from build123d import *

# Parameters (mm, degrees)
F0_R      = 3.7
F0_R_2    = 2.7
F1_DEPTH  = 35
F2_W      = 2
F2_H      = 6.1218521535
F3_DEPTH  = 35.001
F6_W      = 26.1
F6_H      = 2
F8_W      = 26.1
F8_H      = 2
F11_DEPTH = 1.7
F13_DEPTH = 1.7
F14_R     = 6.1
F15_DEPTH = 19.2330509442
F14_R_2   = 8.1
F16_DEPTH = 0.5
F17_R     = 0.49999
F19_DEPTH = 26.1
F21_DEPTH = 1.7
F23_DEPTH = 1.7


# Not quite as in the source:
# - a fillet or chamfer is up to 0.001 mm smaller than in the source, because OpenCascade refuses the exact size


with BuildPart() as f1:
    # F0 (on Top) → F1 (new body)
    with BuildSketch(Plane.XY):
        with Locations((-15.75, 0)):
            Circle(F0_R)
        with Locations((-15.75, 0)):
            Circle(F0_R_2, mode=Mode.SUBTRACT)
    extrude(amount=F1_DEPTH)

    # F2 (on Top) → F3 (cut, through all)
    with BuildSketch(Plane.XY):
        with Locations((-15.75, 2.7)):
            Rectangle(F2_W, F2_H)
    extrude(amount=F3_DEPTH, mode=Mode.SUBTRACT)


with BuildPart() as f5_1:
    # F5: instance of F1
    add(f1.part.mirror(Plane.YZ))


with BuildPart() as f1_1:
    add(f1.part)

    add(f5_1.part)  # F9 merges F5_1
    # F6 (on Top) → F9 section 0
    with BuildSketch(Plane.XY):
        with Locations((0, -10)):
            Rectangle(F6_W, F6_H)
    # F8 (on offset) → F9 section 1
    with BuildSketch(Plane.XY.offset(35)):
        with Locations((0, 10.2072594216)):
            Rectangle(F8_W, F8_H)
    loft()

    # F10 (on face) → F11 (join, through all)
    with BuildSketch(Plane.YZ.offset(13.05)):
        Polygon((2.5079872408, 19.9324185939), (2.5298221281, 19.9702377282), (11.2072594216, 35), (2.5079872408, 35), align=None)
    extrude(amount=F11_DEPTH)

    # F12 (on face) → F13 (join, through all)
    with BuildSketch(Plane(origin=(-13.05, 0, 0), x_dir=(0, -1, 0), z_dir=(-1, 0, 0))):
        Polygon((-11.2072594216, 35), (-2.5298221281, 19.9702377282), (-2.5079872408, 19.9324185939), (-2.5079872408, 35), align=None)
    extrude(amount=F13_DEPTH)

    # F14 (on face) → F15 (cut, through all)
    with BuildSketch(Plane(origin=(0, -8.25, 4.7631397208), x_dir=(1, 0, 0), z_dir=(0, -0.8660254038, 0.5))):
        with Locations((0, 16.5)):
            Circle(F14_R)
    extrude(amount=-F15_DEPTH, mode=Mode.SUBTRACT)

    # F14 (on face) → F16 (join)
    with BuildSketch(Plane(origin=(0, -8.25, 4.7631397208), x_dir=(1, 0, 0), z_dir=(0, -0.8660254038, 0.5))):
        with Locations((0, 16.5)):
            Circle(F14_R_2)
        with Locations((0, 16.5)):
            Circle(F14_R, mode=Mode.SUBTRACT)
    extrude(amount=F16_DEPTH)

    # F17 (radius 0.5 in the source; OpenCascade refuses exactly that, so slightly less here)
    f17_edges = [f1_1.edges().sort_by_distance(p)[0] for p in [
        (-8.1, -0.433013, 19.302559),
    ]]
    fillet(f17_edges, radius=F17_R)

    # F18 (on face) → F19 (cut, through all)
    with BuildSketch(Plane.YZ.offset(13.05)):
        Polygon((-5.3, 9.8726896031), (-11, 0), (-9, 0), (-5.3, 6.408587988), align=None)
    extrude(amount=-F19_DEPTH, mode=Mode.SUBTRACT)

    # F20 (on face) → F21 (join, through all)
    with BuildSketch(Plane.YZ.offset(13.05)):
        Polygon((-2.5298221281, 14.6707784232), (-5.3, 9.8726896031), (-5.3, 6.408587988), (-2.5298221281, 6.408587988), align=None)
    extrude(amount=F21_DEPTH)

    # F22 (on face) → F23 (join, through all)
    with BuildSketch(Plane(origin=(-13.05, 0, 0), x_dir=(0, -1, 0), z_dir=(-1, 0, 0))):
        Polygon((5.3, 6.408587988), (5.3, 9.8726896031), (2.5298221281, 14.6707784232), (2.5298221281, 6.408587988), align=None)
    extrude(amount=F23_DEPTH)


solid = f1_1.part
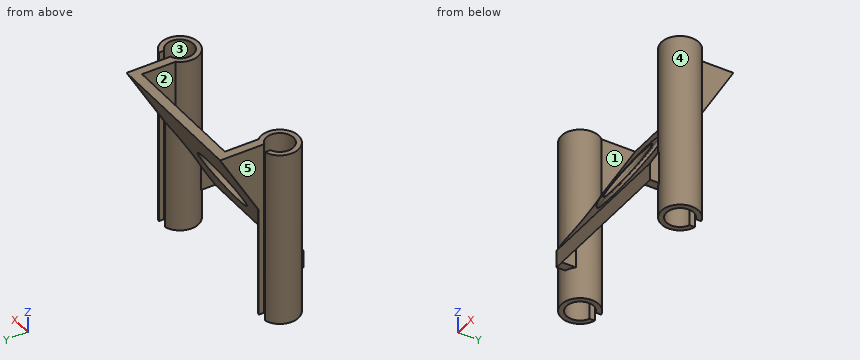
Verification items for the finished model (mm, model axes). Face numbers are marked on the shaded views. A direction names the side the tool comes from. Give positions to 0.01 mm unless a question says otherwise; leave off trailing zeros. Write each loop counter-clockwise with the first axis right and the second up, starting at its lowest first coordinate (ties: lowest second). Pieces come first, ordered by that corner, then holes.
(1) Cross-section at A-A (x = 15.75). Enter the section's corners in (y, z), plus the area to 3 significant figures.
(2) Access from +Z, -Z, +X, -X, +Y, -Y to the whole of each face (thin tool, end or side, straight path). Record for the marked faces 3, 4 and 5.
(3) Cross-section at D-D (x = 10). Enter the section's corners in (y, z), plus the area to 3 significant figures.
(4) Cross-section at B-B (y = 7). Enter the section's corners in (x, z).
(5) Gauge pin test, flat ends, axial feed: pin 1 (5 mm diameter, centred on y = 2, z = 26.5, fed in from -X); pin 2 (0.5 mm diameter, centred on y = -4.5, z = 9.5, fed in from -X); pin 3 (8 mm diameter, centred on x = 1.5, y = 0.5, fed in from -Z); pin 4 (5.5 mm diameter, centred on y = 6, z = 28, fed in from -X). Record the tip position at first contact, or that the pin passes through.
(6) Cross-section at C-C (y = 2). State how many separate pieces and enclosed holes the cut face has, plus the area to 3 significant figures.
(7) Material ranges on line 1 (X direction, y = 0, z = 24); line 2 (X direction, y = 2, z = 24); line 3 (Y direction, x = -14.5, z = 29), recorded low to high.
(8) Mould release check, pull along X, two halves, no side actions. Record for the marked faces 1 and 2: +X half, -X half, draft (parallel to the pull), parting line (faces both ways), or undercut.
Worked out:
1. outline: (-3.7, 0) - (-2.7, 0) - (-2.7, 35) - (-3.7, 35) - close
1. area: 35.0 mm2
2. face 3: +Z, -Z
2. face 4: none
2. face 5: +Z, -Z, +Y
3. outline: (-5.3, 6.41) - (11.21, 35) - (9.21, 35) - (-5.3, 9.87) - close
3. area: 53.7 mm2
4. outline: (-14.75, 27.71) - (14.75, 27.71) - (14.75, 35) - (13.05, 35) - (13.05, 31.18) - (-13.05, 31.18) - (-13.05, 35) - (-14.75, 35) - close
5. pin 1: stops at x = -19.45
5. pin 2: stops at x = -14.75
5. pin 3: stops at z = 9.53
5. pin 4: stops at x = -17.52
6. separate pieces: 4
6. enclosed holes: 0
6. area: 236 mm2
7. line 1: x = -19.45 to -18.45, -13.05 to -12.05, 12.05 to 13.05, 18.45 to 19.45
7. line 2: x = -18.86 to -17.56, -13.94 to -12.64, 12.64 to 13.94, 17.56 to 18.86
7. line 3: y = -3.48 to -2.39, 2.39 to 7.74
8. face 1: undercut
8. face 2: undercut
